Geometry: see drawing. Coordinates: mm, zero at the bounding-box minimum. Give positions to 0.01 mm unless a question says otherwise; leave off trailing zeros. Loops run counter-clockwise (first coordinate to the right, second up) from the corner with the lowest first, then second, coordinate; pieces in that order, holes last. Notation, with made-up numbers: M -17.75,73 L 25.25,73 A30 ccw 25.25,111 Z; hole C 42,-2 d5. An arc over 180 degrees is marked long. Put each result on its own line as item: value.
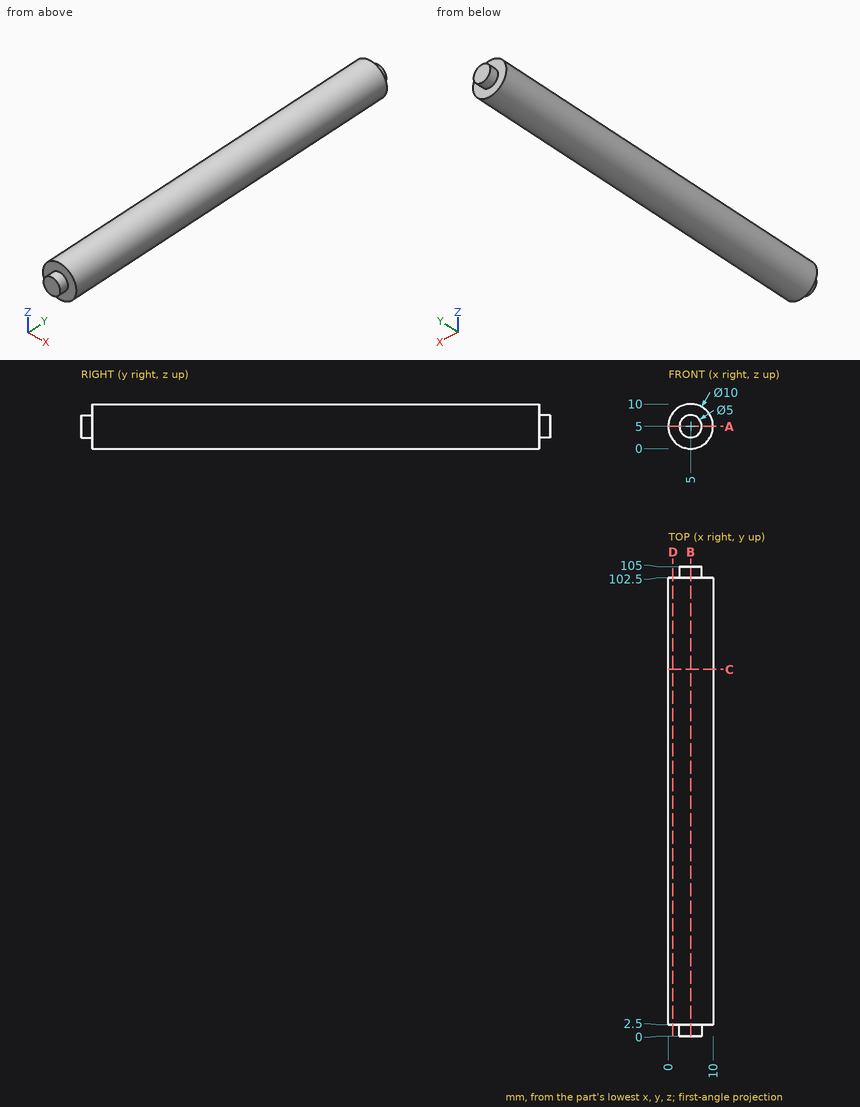
1. Section query D-D (x = 1). Output: boundary loops of the cut face in (y, z), plus the area to 3 significant figures.
Found:
outline: M 2.5,2 L 102.5,2 L 102.5,8 L 2.5,8 Z
area: 600 mm^2
2. Section query C-C (y = 82). Output: boundary loops of the cut face in (x, z).
Found:
outline: C 5,5 d10
3. Section query B-B (x = 5). Output: boundary loops of the cut face in (y, z).
Found:
outline: M 0,2.5 L 2.5,2.5 L 2.5,0 L 102.5,0 L 102.5,2.5 L 105,2.5 L 105,7.5 L 102.5,7.5 L 102.5,10 L 2.5,10 L 2.5,7.5 L 0,7.5 Z
4. Material intervals for line 1 (Y direction, x = 3.75, z = 7.5); line 2 (X direction, y = 72.5, z = 2.25); line 3 (X direction, y = 17, z = 4), sorted ascending. Write a range as from..to.
Found:
line 1: 2.5..102.5
line 2: 0.82..9.18
line 3: 0.1..9.9
5. Section query A-A (z = 5). Output: boundary loops of the cut face in (x, y), plus the area to 4 significant figures.
Found:
outline: M 0,2.5 L 2.5,2.5 L 2.5,0 L 7.5,0 L 7.5,2.5 L 10,2.5 L 10,102.5 L 7.5,102.5 L 7.5,105 L 2.5,105 L 2.5,102.5 L 0,102.5 Z
area: 1,025 mm^2
6. Contact query for flat-ended pins moving along their axis: P1, Ø1, axis at x = 3, y = 67, coming from the -Z side; P2, Ø1, axis at x = 3, z = 7, coming from the -Y side; P3, Ø3, axis at y = 48.5, z = 1.5, coming from the -X side; P4, Ø1, axis at y = 83, z = 8.5, coming from the +X side. Output: stop coordinate, or through.
Found:
P1: z = 0.23
P2: y = 0
P3: x = 0.42
P4: x = 9
